```python
from build123d import *

# Parameters (mm, degrees)
SKETCH1_W           = 6.5
SKETCH1_H           = 40
BOSS_EXTRUDE1_DEPTH = 20
SKETCH2_W           = 15
SKETCH2_H           = 10.1
CUT_EXTRUDE1_DEPTH  = 46.191260217
FILLET1_R           = 2
SKETCH4_W           = 13
SKETCH4_H           = 19.9
CUT_EXTRUDE3_DEPTH  = 46.191260217
SKETCH6_W           = 6.5
SKETCH6_H           = 5
BOSS_EXTRUDE2_DEPTH = 5
FILLET2_R           = 2


with BuildPart() as part:
    # Sketch1 → Boss-Extrude1 (new body)
    with BuildSketch(Plane.XY):
        with Locations((-3.25, 20)):
            Rectangle(SKETCH1_W, SKETCH1_H)
    extrude(amount=BOSS_EXTRUDE1_DEPTH)

    # Sketch2 → Cut-Extrude1 (cut, through all)
    with BuildSketch(Plane(origin=(0, 0, 0), x_dir=(0, 0, -1), z_dir=(1, 0, 0))):
        with Locations((-12.5, 10.05)):
            Rectangle(SKETCH2_W, SKETCH2_H)
    extrude(amount=-CUT_EXTRUDE1_DEPTH, mode=Mode.SUBTRACT)

    # Fillet1
    fillet1_edges = [part.edges().sort_by_distance(p)[0] for p in [
        (-6.5, 15.1, 12.5),
        (-6.5, 10.05, 5),
        (-3.25, 15.1, 5),
        (-6.5, 5, 12.5),
        (-3.25, 5, 5),
        (0, 5, 12.5),
        (0, 10.05, 5),
        (0, 15.1, 12.5),
    ]]
    fillet(fillet1_edges, radius=FILLET1_R)

    # Sketch4 → Cut-Extrude3 (cut, through all)
    with BuildSketch(Plane.ZY.offset(6.5)):
        with Locations((13.5, 30.05)):
            Rectangle(SKETCH4_W, SKETCH4_H)
    extrude(amount=-CUT_EXTRUDE3_DEPTH, mode=Mode.SUBTRACT)

    # Sketch6 → Boss-Extrude2 (add)
    with BuildSketch(Plane(origin=(0, 0, 0), x_dir=(-1, 0, 0), z_dir=(0, 0, -1))):
        with Locations((3.25, 37.5)):
            Rectangle(SKETCH6_W, SKETCH6_H)
    extrude(amount=BOSS_EXTRUDE2_DEPTH)

    # Fillet2
    fillet2_edges = [part.edges().sort_by_distance(p)[0] for p in [
        (-3.25, 0, 20),
        (-6.5, 1.5, 20),
        (-3.25, 5, 20),
        (-0.585786438, 4.414213562, 20),
        (-5.914213562, 4.414213562, 20),
        (0, 18.6, 20),
        (-3.25, 15.1, 20),
        (-0.585786438, 15.685786438, 20),
        (-5.914213562, 15.685786438, 20),
        (0, 1.5, 20),
        (-3.25, 0, 0),
        (0, 17.5, 0),
        (-6.5, 18.6, 20),
        (-6.5, 40, 1),
        (0, 40, 1),
        (0, 20.1, 13.5),
        (-3.25, 20.1, 20),
        (0, 30.05, 7),
        (-3.25, 20.1, 7),
        (-3.25, 40, 7),
        (-6.5, 30.05, 7),
        (-6.5, 20.1, 13.5),
        (-6.5, 17.5, 0),
        (0, 0, 10),
        (-3.25, 35, 0),
        (-6.5, 0, 10),
        (0, 35, -2.5),
        (-6.5, 35, -2.5),
        (0, 37.5, -5),
        (-3.25, 35, -5),
        (-6.5, 37.5, -5),
        (-3.25, 40, -5),
    ]]
    fillet(fillet2_edges, radius=FILLET2_R)


solid = part.part
```
The listing builds one solid part. Answer for the finished solid, in the listing's coordinates (mm). A direction names the side the tool comes from. Coordinates: 2 decimals unless noted, no trailing zeros. Loops run counter-clockwise (first coordinate to the right, second up) from the corner with the lowest first, then second, coordinate; pieces in that order, holes last. Notation, with made-up numbers: (12, 37) -> (46, 37) arc R20 cw to (46, 47) -> close; hole circle Ø1 at (69.25, -30). An arc over 180 degrees is marked (long way). Return JSON: item names as keys, results as strings. Group by question number.
(1) Given pin 1 Ø0.8 at (x, z) = (-3.5, -2.5) entering from -Y; pin 2 Ø3 at (x, y) = (-4, 29.5) entering from +Z; pin 3 Ø3 at (x, y) = (-3, 11.5) entering from +Z, each flat-ended and moving along its own axis, determine where each tip first touches the part or whether it passes through.
(2) Determine the mould class of faces 1 (the cylindrical face through (-5.93, 2.51, 19.4)), 2 (the cylindrical face through (-3.27, 35.6, -4.43)), 3 (the flat face through (-3, 10, 5)) for opening direction Y: released by +Y, released by -Y, zero draft, split by the parting line, or undercut.
(3) A cutting plane is placed at A-A on z = 11.25. Write down the section's boundary in (x, y).
(4) Which of the six approach directions +Z, -Z, +X, -X, +Y, -Y give full straight-line access (tool end or side, diameter ignored) to faces 4 (the cylindrical face through (-0.6, 10.09, 4.43)), 5 (the flat face through (-3, 20.1, 13)), 6 (the cylindrical face through (-5.93, 19.5, 13.56))?
(5) A cutting plane is placed at B-B on y = 8. Write down the section's boundary in (x, z).
(6) Find the intervals of material crossed by probe 1 along Y at (x, z) = (-3.75, 13); probe 2 along Z at (x, y) = (-2.75, 31); probe 3 along Y at (x, z) = (-1, 17), in increasing order. Write a range as from..to.
(7) A cutting plane is placed at C-C on x = -3.75. Write down the section's boundary in (y, z).
(8) A cutting plane is placed at D-D on y = 23.5. Write down the section's boundary in (x, z).
The answers:
{
 "1": {"pin 1": "stops at y = 35", "pin 2": "stops at z = 7", "pin 3": "stops at z = 5"},
 "2": {"face 1": "zero draft", "face 2": "released by -Y", "face 3": "undercut"},
 "3": {"outline": "(-6.5, 2) arc R2 ccw to (-4.5, 0) -> (-2, 0) arc R2 ccw to (0, 2) -> (0, 3) arc R2 ccw to (-2, 5) -> (-4.5, 5) arc R2 ccw to (-6.5, 3) -> close; (-6.5, 17.1) arc R2 ccw to (-4.5, 15.1) -> (-2, 15.1) arc R2 ccw to (0, 17.1) -> (0, 18.1) arc R2 ccw to (-2, 20.1) -> (-4.5, 20.1) arc R2 ccw to (-6.5, 18.1) -> close"},
 "4": {"face 4": "+Z, +X", "face 5": "+Z, +X, -X, +Y", "face 6": "+Z, -X, +Y"},
 "5": {"outline": "(-6.5, 2) arc R2 ccw to (-4.5, 0) -> (-2, 0) arc R2 ccw to (0, 2) -> (0, 3) arc R2 ccw to (-2, 5) -> (-4.5, 5) arc R2 ccw to (-6.5, 3) -> close"},
 "6": {"probe 1": "y = 0..5, 15.1..20.1", "probe 2": "z = 0..7", "probe 3": "y = 0.27..4.73, 15.37..19.83"},
 "7": {"outline": "(0, 2) arc R2 ccw to (2, 0) -> (33, 0) arc R2 cw to (35, -2) -> (35, -3) arc R2 ccw to (37, -5) -> (38, -5) arc R2 ccw to (40, -3) -> (40, 5) arc R2 ccw to (38, 7) -> (22.1, 7) arc R2 cw to (20.1, 9) -> (20.1, 18) arc R2 ccw to (18.1, 20) -> (17.1, 20) arc R2 ccw to (15.1, 18) -> (15.1, 7) arc R2 cw to (13.1, 5) -> (7, 5) arc R2 cw to (5, 7) -> (5, 18) arc R2 ccw to (3, 20) -> (2, 20) arc R2 ccw to (0, 18) -> close"},
 "8": {"outline": "(-6.5, 2) arc R2 ccw to (-4.5, 0) -> (-2, 0) arc R2 ccw to (0, 2) -> (0, 5) arc R2 ccw to (-2, 7) -> (-4.5, 7) arc R2 ccw to (-6.5, 5) -> close"}
}
